Check sheet for the modelled part. Datum: model origin and axes. Units: mm. A direction names the side the tool comes from. Give positions to 0.01 mm unless a question says otherwise; leave off trailing zeros. Write each loop counter-clockwise with the first axis right and the second up, starting at its lowest first coordinate (ties: lowest second). Pieces come first, ordered by that corner, then holes. Notation, with made-up numbers: M 62.25,83.5 L 115.25,83.5 A25 ccw 115.25,99.5 Z; hole C -38,60 d2. An arc over 180 degrees is marked long. Write each question's results on one line, items separated by ' | '. Start each with the question number.
from build123d import *

# Parameters (mm, degrees)
CROQUIS1_R              = 1.75
SALIENTE_EXTRUIR1_DEPTH = 8.5
REDONDEO1_R             = 3
CORTAR_EXTRUIR1_START   = -6
CROQUIS2_R              = 1.5
CORTAR_EXTRUIR1_DEPTH   = 6


with BuildPart() as part:
    # Croquis1 → Saliente-Extruir1 (new body)
    with BuildSketch(Plane.XY):
        Polygon((1, 0), (-1, 0), (-1, 20), (-3, 20), (-3, -5.5), (3, -5.5), (3, 20), (1, 20), align=None)
        with Locations((0, -2.75)):
            Circle(CROQUIS1_R, mode=Mode.SUBTRACT)
    extrude(amount=SALIENTE_EXTRUIR1_DEPTH)

    # Redondeo1
    redondeo1_edges = [part.edges().sort_by_distance(p)[0] for p in [
        (-3, -5.5, 4.25),
        (3, -5.5, 4.25),
    ]]
    fillet(redondeo1_edges, radius=REDONDEO1_R - 0.0001)  # a hair under: the kernel refuses the full size

    # Croquis2 → Cortar-Extruir1 (cut)
    with BuildSketch(Plane(origin=(3, 0, 0), x_dir=(0, 0, -1), z_dir=(1, 0, 0)).offset(CORTAR_EXTRUIR1_START)):
        with Locations(Location((-4.25, 16, 0), (0, 0, 90))):
            Circle(CROQUIS2_R)
        with Locations(Location((-4.25, 4, 0), (0, 0, 90))):
            Circle(CROQUIS2_R)
    extrude(amount=CORTAR_EXTRUIR1_DEPTH, mode=Mode.SUBTRACT)


solid = part.part
Q1. Scan lines: L1, parallel to Z at x = -2.2, y = 16; L2, parallel to X at y = 17.5, z = 7; L3, parallel to Y at x = 1.5, z = 4.25. Record each from-to range of solid material in increasing order.
Q2. Section check D-D on x = 0.25. Record the boundary of the cut face in (y, z), plus the area to 3 significant figures.
Q3. Section check A-A on z = 4.25. State how many separate pieces and enclosed holes the cut face has, plus the area to 3 significant figures.
Q4. Depth check by flat-ended pin: pin 1 Ø1 at (x, z) = (1, 4.5) entering from -Y; pin 2 Ø1.6 at (x, z) = (0, 3.5) entering from +Y. Enter the tip coordinate at first touch or a pass-through.
Q5. Release check for a two-part mould opening along Y. For faces 1 (the face through (-2.14, -4.6, 4.31)), 2 (the face through (1.986, 5.386, 3.675)), 3 (the face through (1.3, 7.4, 0)) record: pulls with the +Y half, pulls with the -Y half, needs draft (parallel to the pull), parting line crosses it, or undercut.
Q6. Tool access check on faces 4 (the face through (-3, 9, 4)), 5 (the face through (-1, 10, 4)). Record the directions out of +Z, -Z, +X, -X, +Y, -Y that give a thin tool (end or side, any length) a straight path to the whole face; none if there is none.
Q7. Section check C-C on y = 6.5. Record the boundary of the cut face in (x, z).
Q8. Section check B-B on y = 16. Record the boundary of the cut face in (x, z), plus the area to 3 significant figures.
Check result:
1) L1: 0 to 2.75, 5.75 to 8.5 | L2: -3 to -1, 1 to 3 | L3: -5.1 to -3.65, -1.85 to 2.5, 5.5 to 14.5, 17.5 to 20
2) outline: M -5.49,0 L -4.48,0 L -4.48,8.5 L -5.49,8.5 Z; M -1.02,0 L 0,0 L 0,8.5 L -1.02,8.5 Z | area: 17.2 mm^2
3) separate pieces: 5 | enclosed holes: 1 | area: 75.5 mm^2
4) pin 1: y = -5.46 | pin 2: y = 0
5) face 1: pulls with the -Y half | face 2: undercut | face 3: needs draft
6) face 4: +Z, -Z, -X, +Y, -Y | face 5: +Z, -Z, +Y
7) outline: M -3,0 L -1,0 L -1,8.5 L -3,8.5 Z; M 1,0 L 3,0 L 3,8.5 L 1,8.5 Z
8) outline: M -3,0 L -1,0 L -1,2.75 L -3,2.75 Z; M -3,5.75 L -1,5.75 L -1,8.5 L -3,8.5 Z; M 1,0 L 3,0 L 3,2.75 L 1,2.75 Z; M 1,5.75 L 3,5.75 L 3,8.5 L 1,8.5 Z | area: 22.0 mm^2
